Build history of the part. All positions in model axes, mm. Round coordinates to 2 decimals unless told otherwise and drop trailing zeros. Order: outer loops, then holes, each group sorted by start corner. A loop starts at its lowest first (then second) coordinate and runs counter-clockwise, first axis right, second up. Notation, with made-up numbers: (4, 57.25) -> (25, 57.25) arc R12 cw to (25, 74.25) -> close; hole circle Ø10 at (27, 20.25). An arc over 180 degrees is marked (long way). Write item = value, one per line.
from build123d import *

# Parameters (mm, degrees)
SKETCH1_W           = 212
SKETCH1_H           = 76
BOSS_EXTRUDE1_DEPTH = 50
CUT_EXTRUDE1_DEPTH  = 77
SKETCH4_R           = 2.5
CUT_EXTRUDE2_DEPTH  = 77
FILLET1_R           = 4


with BuildPart() as part:
    # Sketch1 → Boss-Extrude1 (new body)
    with BuildSketch(Plane(origin=(0, 0, 0), x_dir=(1, 0, 0), z_dir=(0, 1, 0))):
        Rectangle(SKETCH1_W, SKETCH1_H)
    extrude(amount=BOSS_EXTRUDE1_DEPTH)

    # Sketch2 → Cut-Extrude1 (cut)
    with BuildSketch(Plane.XY.offset(38)):
        Polygon((101, 0), (100, 45), (88.181819, 45), (87.181819, 0), align=None)
        Polygon((68.363638, 0), (82.181819, 0), (81.181819, 45), (69.363638, 45), align=None)
        Polygon((49.545457, 0), (63.363638, 0), (62.363638, 45), (50.545457, 45), align=None)
        Polygon((30.727276, 0), (44.545457, 0), (43.545457, 45), (31.727276, 45), align=None)
        Polygon((11.909095, 0), (25.727276, 0), (24.727276, 45), (12.909095, 45), align=None)
        Polygon((-6.909086, 0), (6.909095, 0), (5.909095, 45), (-5.909086, 45), align=None)
        Polygon((-25.727267, 0), (-11.909086, 0), (-12.909086, 45), (-24.727267, 45), align=None)
        Polygon((-44.545448, 0), (-30.727267, 0), (-31.727267, 45), (-43.545448, 45), align=None)
        Polygon((-63.363629, 0), (-49.545448, 0), (-50.545448, 45), (-62.363629, 45), align=None)
        Polygon((-82.18181, 0), (-68.363629, 0), (-69.363629, 45), (-81.18181, 45), align=None)
        Polygon((-100.999991, 0), (-87.18181, 0), (-88.18181, 45), (-99.999991, 45), align=None)
    extrude(amount=-CUT_EXTRUDE1_DEPTH, mode=Mode.SUBTRACT)

    # Sketch4 → Cut-Extrude2 (cut)
    with BuildSketch(Plane(origin=(0, 50, 0), x_dir=(1, 0, 0), z_dir=(0, 1, 0))):
        with Locations((-96, 25.5)):
            Circle(SKETCH4_R)
        with Locations((-96, -25.5)):
            Circle(SKETCH4_R)
        with Locations((96, 25.5)):
            Circle(SKETCH4_R)
        with Locations((96, -25.5)):
            Circle(SKETCH4_R)
        with Locations((-56, 8)):
            Circle(SKETCH4_R)
        with Locations((-20, 8)):
            Circle(SKETCH4_R)
        with Locations((-20, -8)):
            Circle(SKETCH4_R)
        with Locations((-56, -8)):
            Circle(SKETCH4_R)
        with Locations((56, -8)):
            Circle(SKETCH4_R)
        with Locations((20, -8)):
            Circle(SKETCH4_R)
        with Locations((20, 8)):
            Circle(SKETCH4_R)
        with Locations((56, 8)):
            Circle(SKETCH4_R)
    extrude(amount=-CUT_EXTRUDE2_DEPTH, mode=Mode.SUBTRACT)

    # Fillet1
    fillet1_edges = [part.edges().sort_by_distance(p)[0] for p in [
        (106, 25, 38),
        (-106, 25, 38),
        (-106, 25, -38),
        (106, 25, -38),
    ]]
    fillet(fillet1_edges, radius=FILLET1_R)


solid = part.part
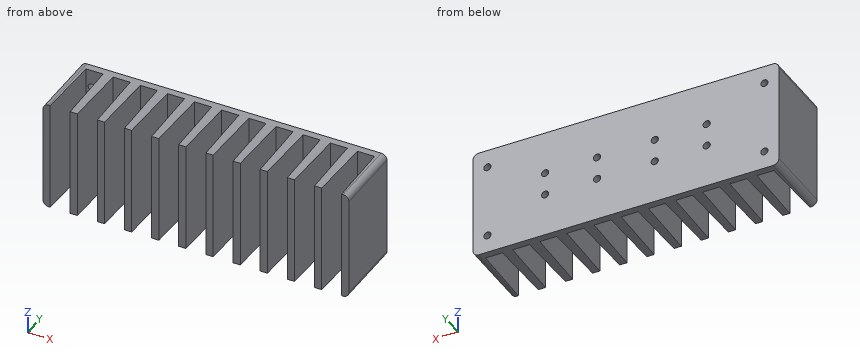
Q1. Cut at D-D, the plane x = 76.5. List the corners of the cut face in (y, z).
Check values:
outline = (45, -38) -> (50, -38) -> (50, 38) -> (45, 38) -> close
Q2. Probe probe 1 along Z at (x, y) = (96, 48); probe 2 along X at (y, z) = (46.35, 8); probe 3 along Y at (x, z) = (61.5, -28.5). List the from-to ranges inside material, lowest first.
Check values:
probe_1 = -38 to -28, -23 to 23, 28 to 38
probe_2 = -106 to -58.5, -53.5 to -22.5, -17.5 to 17.5, 22.5 to 53.5, 58.5 to 106
probe_3 = 45 to 50
Q3. Flat gauge pins, fed straight in: pin 1 (8 mm diameter, centred on x = 6, y = 14.5, fed in from -Z); pin 2 (9.5 mm diameter, centred on x = -56.5, z = 14.5, fed in from -Y). Where does each tip first touch, or does it go through?
Check values:
pin_1 = -38
pin_2 = 45
Q4. Cut at B-B, the plane z = -8. Give the number of separate pieces and of enclosed holes in the cut face, and give its area (4 significant figures).
Check values:
separate_pieces = 5
enclosed_holes = 0
area = 4,155 mm²
Q5. Cut at A-A, the plane x = 20. List the corners of the cut face in (y, z), and give its area (3 significant figures).
Check values:
outline = (45, -38) -> (50, -38) -> (50, -10.5) -> (45, -10.5) -> close; (45, -5.5) -> (50, -5.5) -> (50, 5.5) -> (45, 5.5) -> close; (45, 10.5) -> (50, 10.5) -> (50, 38) -> (45, 38) -> close
area = 330 mm²
